```python
from build123d import *

# Parameters (mm, degrees)
SKETCH1_W            = 41
SKETCH1_H            = 20
BOSS_EXTRUDE1_DEPTH  = 40
CHAMFER1_SIZE        = 2
SKETCH2_R            = 2.25
CUT_EXTRUDE1_DEPTH   = 1
SKETCH3_W            = 19
SKETCH3_H            = 2.5
BOSS_EXTRUDE2_DEPTH  = 7
FILLET1_R            = 1.5
SKETCH4_W            = 7
SKETCH4_H            = 1
BOSS_EXTRUDE3_DEPTH  = 1.5
CUT_EXTRUDE2_DEPTH   = 1
SKETCH6_R            = 2
CUT_EXTRUDE3_DEPTH   = 2.5
FILLET1_OF_MIRROR1_R = 1.5
SKETCH7_W            = 41
SKETCH7_H            = 20
CUT_EXTRUDE4_DEPTH   = 3
SKETCH8_W            = 40
SKETCH8_H            = 19
BOSS_EXTRUDE4_DEPTH  = 0.5
BOSS_EXTRUDE6_DEPTH  = 2.5
SKETCH10_W           = 11
SKETCH10_H           = 16
BOSS_EXTRUDE7_DEPTH  = 0.5
SKETCH11_R           = 6.5
BOSS_EXTRUDE8_DEPTH  = 1.5
SKETCH12_R           = 5.5
BOSS_EXTRUDE9_DEPTH  = 0.5
SKETCH13_R           = 3
BOSS_EXTRUDE10_DEPTH = 4
SKETCH14_R           = 1
CUT_EXTRUDE5_DEPTH   = 8
SKETCH15_W           = 7
SKETCH15_H           = 4
BOSS_EXTRUDE11_DEPTH = 5
SKETCH16_W           = 7
SKETCH16_H           = 4
SKETCH16_W_2         = 6
SKETCH16_H_2         = 3
CUT_EXTRUDE6_DEPTH   = 4
CUT_EXTRUDE7_DEPTH   = 3
CUT_EXTRUDE8_DEPTH   = 7


with BuildPart() as part:
    # Sketch1 → Boss-Extrude1 (new body)
    with BuildSketch(Plane(origin=(0, 0, 0), x_dir=(1, 0, 0), z_dir=(0, 1, 0))):
        Rectangle(SKETCH1_W, SKETCH1_H)
    extrude(amount=BOSS_EXTRUDE1_DEPTH)

    # Chamfer1
    chamfer1_edges = [part.edges().sort_by_distance(p)[0] for p in [
        (0, 0, 10),
        (-20.5, 0, 0),
        (0, 0, -10),
        (20.5, 0, 0),
    ]]
    chamfer(chamfer1_edges, length=CHAMFER1_SIZE)

    # Sketch2 → Cut-Extrude1 (cut)
    with BuildSketch(Plane.XZ):
        with Locations((18.25, 7.75)):
            Circle(SKETCH2_R)
        with Locations((-18.25, 7.75)):
            Circle(SKETCH2_R)
        with Locations((-18.25, -7.75)):
            Circle(SKETCH2_R)
        with Locations((18.25, -7.75)):
            Circle(SKETCH2_R)
    extrude(amount=-CUT_EXTRUDE1_DEPTH, mode=Mode.SUBTRACT)

    # Sketch3 → Boss-Extrude2 (add)
    with BuildSketch(Plane(origin=(20.5, 0, 0), x_dir=(0, 0, -1), z_dir=(1, 0, 0))):
        with Locations((0, 30.75)):
            Rectangle(SKETCH3_W, SKETCH3_H)
    boss_extrude2 = extrude(amount=BOSS_EXTRUDE2_DEPTH)

    # Fillet1
    fillet1_edges = [part.edges().sort_by_distance(p)[0] for p in [
        (27.5, 30.75, 9.5),
        (27.5, 30.75, -9.5),
    ]]
    fillet(fillet1_edges, radius=FILLET1_R)

    # Sketch4 → Boss-Extrude3 (add)
    with BuildSketch(Plane(origin=(0, 32, 0), x_dir=(1, 0, 0), z_dir=(0, 1, 0))):
        with Locations((24, 0)):
            Rectangle(SKETCH4_W, SKETCH4_H)
    boss_extrude3 = extrude(amount=BOSS_EXTRUDE3_DEPTH)

    # Sketch5 → Cut-Extrude2 (cut)
    with BuildSketch(Plane.XY.offset(0.5)):
        Polygon((27.5, 33.5), (27.5, 32), (20.5, 33.5), align=None)
    cut_extrude2 = extrude(amount=-CUT_EXTRUDE2_DEPTH, mode=Mode.SUBTRACT)

    # Sketch6 → Cut-Extrude3 (cut)
    with BuildSketch(Plane(origin=(0, 32, 0), x_dir=(1, 0, 0), z_dir=(0, 1, 0))):
        with Locations((25.6, 5)):
            Circle(SKETCH6_R)
        with Locations((25.6, -5)):
            Circle(SKETCH6_R)
    cut_extrude3 = extrude(amount=-CUT_EXTRUDE3_DEPTH, mode=Mode.SUBTRACT)

    # Mirror1: Boss-Extrude2, Boss-Extrude3, Cut-Extrude2, Cut-Extrude3 across plane
    add(boss_extrude2.mirror(Plane(origin=(0, 0, 0), x_dir=(0, 0, 1), z_dir=(1, 0, 0))))
    add(boss_extrude3.mirror(Plane(origin=(0, 0, 0), x_dir=(0, 0, 1), z_dir=(1, 0, 0))))
    add(cut_extrude2.mirror(Plane(origin=(0, 0, 0), x_dir=(0, 0, 1), z_dir=(1, 0, 0))), mode=Mode.SUBTRACT)
    add(cut_extrude3.mirror(Plane(origin=(0, 0, 0), x_dir=(0, 0, 1), z_dir=(1, 0, 0))), mode=Mode.SUBTRACT)

    # Fillet1 of Mirror1
    fillet1_of_mirror1_edges = [part.edges().sort_by_distance(p)[0] for p in [
        (-27.5, 30.75, 9.5),
        (-27.5, 30.75, -9.5),
    ]]
    fillet(fillet1_of_mirror1_edges, radius=FILLET1_OF_MIRROR1_R)

    # Sketch7 → Cut-Extrude4 (cut)
    with BuildSketch(Plane(origin=(0, 40, 0), x_dir=(1, 0, 0), z_dir=(0, 1, 0))):
        Rectangle(SKETCH7_W, SKETCH7_H)
    extrude(amount=-CUT_EXTRUDE4_DEPTH, mode=Mode.SUBTRACT)

    # Sketch8 → Boss-Extrude4 (add)
    with BuildSketch(Plane(origin=(0, 37, 0), x_dir=(1, 0, 0), z_dir=(0, 1, 0))):
        Rectangle(SKETCH8_W, SKETCH8_H)
    extrude(amount=BOSS_EXTRUDE4_DEPTH)

    # Sketch9 → Boss-Extrude6 (add)
    with BuildSketch(Plane(origin=(0, 37, 0), x_dir=(1, 0, 0), z_dir=(0, 1, 0))):
        with BuildLine():
            Line((6.141101056, 9), (-14.5, 9))
            Line((-14.5, 9), (-14.5, 5))
            ThreePointArc((-14.5, 5), (-16.5, 0), (-14.5, -5))
            Line((-14.5, -5), (-14.5, -9))
            Line((-14.5, -9), (6.141101056, -9))
            ThreePointArc((6.141101056, -9), (20.5, 0), (6.141101056, 9))
        make_face()
    extrude(amount=BOSS_EXTRUDE6_DEPTH)

    # Sketch10 → Boss-Extrude7 (add)
    with BuildSketch(Plane(origin=(0, 39.5, 0), x_dir=(1, 0, 0), z_dir=(0, 1, 0))):
        with BuildLine():
            Line((-14.5, 9), (-1.5, 9))
            Line((-1.5, 9), (-1.5, 2))
            ThreePointArc((-1.5, 2), (0.5, 0), (-1.5, -2))
            Line((-1.5, -2), (-1.5, -9))
            Line((-1.5, -9), (-14.5, -9))
            Line((-14.5, -9), (-14.5, 9))
        make_face()
        with Locations((-8, 0)):
            Rectangle(SKETCH10_W, SKETCH10_H, mode=Mode.SUBTRACT)
    extrude(amount=BOSS_EXTRUDE7_DEPTH)

    # Sketch11 → Boss-Extrude8 (add)
    with BuildSketch(Plane(origin=(0, 39.5, 0), x_dir=(1, 0, 0), z_dir=(0, 1, 0))):
        with Locations((10.5, 0)):
            Circle(SKETCH11_R)
    extrude(amount=BOSS_EXTRUDE8_DEPTH)

    # Sketch12 → Boss-Extrude9 (add)
    with BuildSketch(Plane(origin=(0, 41, 0), x_dir=(1, 0, 0), z_dir=(0, 1, 0))):
        with Locations((10.5, 0)):
            Circle(SKETCH12_R)
    extrude(amount=BOSS_EXTRUDE9_DEPTH)

    # Sketch13 → Boss-Extrude10 (add)
    with BuildSketch(Plane(origin=(0, 41.5, 0), x_dir=(1, 0, 0), z_dir=(0, 1, 0))):
        with Locations((10.5, 0)):
            Circle(SKETCH13_R)
    extrude(amount=BOSS_EXTRUDE10_DEPTH)

    # Sketch14 → Cut-Extrude5 (cut)
    with BuildSketch(Plane(origin=(0, 45.5, 0), x_dir=(1, 0, 0), z_dir=(0, 1, 0))):
        with Locations((10.5, 0)):
            Circle(SKETCH14_R)
    extrude(amount=-CUT_EXTRUDE5_DEPTH, mode=Mode.SUBTRACT)

    # Sketch15 → Boss-Extrude11 (add)
    with BuildSketch(Plane(origin=(20.5, 0, 0), x_dir=(0, 0, -1), z_dir=(1, 0, 0))):
        with Locations((0, 6.5)):
            Rectangle(SKETCH15_W, SKETCH15_H)
    extrude(amount=BOSS_EXTRUDE11_DEPTH)

    # Sketch16 → Cut-Extrude6 (cut)
    with BuildSketch(Plane(origin=(25.5, 0, 0), x_dir=(0, 0, -1), z_dir=(1, 0, 0))):
        with Locations((0, 6.5)):
            Rectangle(SKETCH16_W, SKETCH16_H)
        with Locations((0, 6.5)):
            Rectangle(SKETCH16_W_2, SKETCH16_H_2, mode=Mode.SUBTRACT)
    extrude(amount=-CUT_EXTRUDE6_DEPTH, mode=Mode.SUBTRACT)

    # Sketch17 → Cut-Extrude7 (cut)
    with BuildSketch(Plane.XZ.offset(-5)):
        Polygon((21.5, 3), (25.5, 2.5), (25.5, 3), align=None)
        Polygon((21.5, -3), (25.5, -2.5), (25.5, -3), align=None)
    extrude(amount=-CUT_EXTRUDE7_DEPTH, mode=Mode.SUBTRACT)

    # Sketch18 → Cut-Extrude8 (cut)
    with BuildSketch(Plane(origin=(0, 0, -3.5), x_dir=(-1, 0, 0), z_dir=(0, 0, -1))):
        Polygon((-21.5, 8), (-25.5, 8), (-25.5, 7.5), align=None)
        Polygon((-21.5, 5), (-25.5, 5), (-25.5, 5.5), align=None)
    extrude(amount=-CUT_EXTRUDE8_DEPTH, mode=Mode.SUBTRACT)


solid = part.part
```
Input: part model. Units: mm. Frame: model coordinates. A direction names the side the tool comes from. Give positions to 0.01 mm unless a question says otherwise; leave off trailing zeros. Write each loop counter-clockwise with the first axis right and the second up, starting at its lowest first coordinate (ties: lowest second). Pieces come first, ordered by that corner, then holes. Notation, with made-up numbers: (57.5, 17) - (72.5, 17) arc R18 ccw to (72.5, 37) - close; hole circle Ø4 at (-9, 33.25). An arc over 180 degrees is marked (long way). Write item = value, one per line. Start each with the question number.
1. Section query C-C, the plane y = 38.5. Output: boundary loops of the cut face in (x, z), then the cut area to 3 significant figures.
2. Mould query, pull axis Y, two halves, no side actions, for faces 6 (the flat face through (18, 1, 7)), 7 (the flat face through (18, 37.5, -8)), 8 (the flat face through (23, 29.5, 0)). Classes: released by +Y, released by -Y, zero draft, split by the parting line, or undercut.
3. Section query B-B, the plane x = -7. Output: boundary loops of the cut face in (y, z).
4. Ray query, L1, parallel to Z at x = 25.6, y = 30.7; L2, parallel to Z at x = -25, y = 30; L3, parallel to Y at x = 5, z = 7. Return the intervals inside material, ascending.
5. Section query A-A, the plane y = 30.5. Output: boundary loops of the cut face in (x, z).
6. Section query D-D, the plane x = -21.5. Output: boundary loops of the cut face in (y, z), then the cut area to 3 significant figures.
7. First-contact query: pin 1 Ø2 at (x, y) = (-23.5, 31) entering from +Z; pin 2 Ø1 at (y, z) = (14.5, -6) entering from -X; pin 3 Ø5.5 at (x, z) = (-0.5, 2.5) entering from +Y. Flat tips, straight axial feed; report the tip coordinate or a pass-through.
8. Access query for faces 1 (the flat face through (-14.5, 39.8, 0.1)), 2 (the flat face through (-15, 39.5, 0)), 3 (the flat face through (23.528, 7.746, -0.042)), 4 (the cylindrical face through (20.496, 38.232, 0.283)), 5 (the flat face through (-23, 29.5, 0)). Directions: +Z, -Z, +X, -X, +Y, -Y. A direction counts if a zero-diameter tool reaches every point of the face in a straight line with its end or side. Return the directions, or none.
Check sheet entries:
q1.outline = (-14.5, -9) - (6.14, -9) arc R10 ccw (long way) to (6.14, 9) - (-14.5, 9) - (-14.5, 5) arc R7.25 ccw to (-14.5, -5) - close; hole circle Ø2 at (10.5, 0)
q1.area = 624 mm2
q2.face_6 = released by -Y
q2.face_7 = released by +Y
q2.face_8 = undercut
q3.outline = (0, -8) - (2, -10) - (37, -10) - (37, -9.5) - (37.5, -9.5) - (37.5, -9) - (40, -9) - (40, -8) - (39.5, -8) - (39.5, 8) - (40, 8) - (40, 9) - (37.5, 9) - (37.5, 9.5) - (37, 9.5) - (37, 10) - (2, 10) - (0, 8) - close
q4.L1 = -9.5 to -7, -3 to 3, 7 to 9.5
q4.L2 = -9.5 to -6.91, -3.09 to 3.09, 6.91 to 9.5
q4.L3 = 0 to 39.5
q5.outline = (-27.5, -8) arc R1.5 ccw to (-26, -9.5) - (-20.5, -9.5) - (-20.5, -10) - (20.5, -10) - (20.5, -9.5) - (26, -9.5) arc R1.5 ccw to (27.5, -8) - (27.5, -5.62) arc R2 cw (long way) to (27.5, -4.38) - (27.5, 4.38) arc R2 cw (long way) to (27.5, 5.62) - (27.5, 8) arc R1.5 ccw to (26, 9.5) - (20.5, 9.5) - (20.5, 10) - (-20.5, 10) - (-20.5, 9.5) - (-26, 9.5) arc R1.5 ccw to (-27.5, 8) - (-27.5, 5.62) arc R2 cw (long way) to (-27.5, 4.38) - (-27.5, -4.38) arc R2 cw (long way) to (-27.5, -5.62) - close
q6.outline = (29.5, -9.5) - (32, -9.5) - (32, -0.5) - (33.29, -0.5) - (33.29, 0.5) - (32, 0.5) - (32, 9.5) - (29.5, 9.5) - close
q6.area = 48.8 mm2
q7.pin_1 = 9.5
q7.pin_2 = -20.5
q7.pin_3 = 40
q8.face_1 = -X, +Y
q8.face_2 = +Z, -Z, -X, +Y
q8.face_3 = +Z, -Z, +X
q8.face_4 = +Y
q8.face_5 = +Z, -Z, -X, -Y
